Work out the finished part from the listing and answer in its coordinate system (mm). Coordinates: 2 decimals unless noted, no trailing zeros. Loops run counter-clockwise (first coordinate to the right, second up) from the corner with the lowest first, then second, coordinate; pieces in that order, holes last. Notation, with made-up numbers: (7.5, 50.25) - (56.5, 50.25) arc R24 cw to (56.5, 76.25) - close; hole circle Ø9 at (7.5, 23.25). An arc over 180 degrees is marked (long way). Write each question's results on one line, items separated by ' | '. Start each with the question number.
1. A cutting plane is placed at B-B on z = 2. Determine the outline of the cut face in (x, y), then the cut area to 3 significant figures.
2. Determine the mould class of faces 1 (the cylindrical face through (53.2, 0.51, 19.06)), 2 (the flat face through (-28, 1, -1)), 3 (the cylindrical face through (-41.89, 0.51, 35.91)), 4 (the cylindrical face through (-62, 0.51, 19.52)) for opening direction X: released by +X, released by -X, zero draft, split by the parting line, or undercut.
3. Each of these flat-tipped pins is pushed along its axis until it touches: P1, Ø5, axis at x = 12, z = -55, coming from the -Y side; P2, Ø3, axis at x = -41.63, z = 37.89, coming from the +Y side. Where does it stop, or does it pass through?
4. A cutting plane is placed at A-A on x = 0. Determine the outline of the cut face in (y, z).
5. A cutting plane is placed at D-D on y = 0.15. State how many separate pieces and enclosed holes the cut face has, then the cut area to 3 significant figures.
6. Find the intervals of material crossed by line 1 along Z through (x, y) = (-12, 0.5); line 2 along X through (y, z) = (0.85, 16.5); line 3 along X through (y, z) = (0.4, -55), in increasing order. Write a range as [from, to].
7. A cutting plane is placed at C-C on z = 27.5. Determine the outline of the cut face in (x, y).
Autodesk Inventor part; units mm, degrees
ref_plane "YZ Plane" through (0, 0, 0) normal (1, 0, 0) x (0, 1, 0)
ref_plane "XZ Plane" through (0, 0, 0) normal (0, 1, 0) x (-1, 0, 0)
ref_plane "XY Plane" through (0, 0, 0) normal (0, 0, 1) x (1, 0, 0)
sketch "Sketch1" plane through (0, 0, 0) normal (0, 0, 1) x (1, 0, 0)
  line L0 (0, 0) -> (-65, 0)
  line L1 (-65, 0) -> (-65, 1)
  line L2 (-65, 1) -> (0, 1)
  line L3 (0, 1) -> (0, 0)
  dimension "baffle_or" = 65
  dimension "d1" = 1
revolve "Revolution1" add sketch "Sketch1" angle 360 about axis through (0, 1, 0) along (0, -1, 0)
sketch "Sketch2" plane through (0, 1, 0) normal (0, 1, 0) x (1, 0, 0)
  circle A0 centre (0, 0) radius 22.5
  dimension "d3" = 45
extrude "Extrusion1" cut sketch "Sketch2" against normal through all
sketch "Sketch3" plane through (0, 1, 0) normal (0, 1, 0) x (1, 0, 0)
  circle A0 centre (0, 55) radius 6.5
  circle A1 centre (-12, 55) radius 2
  circle A2 centre (12, 55) radius 2
  point P0 (0, 0)
  dimension "d12" = 13
  dimension "tubes_r" = 55
  dimension "d14" = 4
  dimension "d15" = 12
  dimension "d16" = 4
  dimension "d17" = 12
extrude "Extrusion2" cut sketch "Sketch3" against normal through all
pattern_circular "Circular Pattern1" count 3 over 360 about axis through (0, 1, 0) along (0, -1, 0) of "Extrusion2"
equation "\"d17\" = d15"
properties part number "Baffle"
Values:
1) outline: (-64.97, 0) - (-22.41, 0) - (-22.41, 1) - (-64.97, 1) - close; (22.41, 0) - (64.97, 0) - (64.97, 1) - (22.41, 1) - close | area: 85.1 mm^2
2) face 1: undercut | face 2: zero draft | face 3: undercut | face 4: split by the parting line
3) P1: y = 0 | P2: through
4) outline: (0, -65) - (1, -65) - (1, -61.5) - (0, -61.5) - close; (0, -48.5) - (1, -48.5) - (1, -22.5) - (0, -22.5) - close; (0, 22.5) - (1, 22.5) - (1, 65) - (0, 65) - close
5) separate pieces: 1 | enclosed holes: 10 | area: 11,200 mm^2
6) line 1: [-63.88, -57], [-53, -19.03], [19.03, 63.88] | line 2: [-62.87, -55.54], [-51.73, -15.3], [15.3, 51.73], [55.54, 62.87] | line 3: [-34.64, -14], [-10, -6.5], [6.5, 10], [14, 34.64]
7) outline: (-58.9, 0) - (-54.13, 0) - (-54.13, 1) - (-58.9, 1) - close; (-41.13, 0) - (41.13, 0) - (41.13, 1) - (-41.13, 1) - close; (54.13, 0) - (58.9, 0) - (58.9, 1) - (54.13, 1) - close
